from build123d import *

# Parameters (mm, degrees)
BOSS_EXTRUDE1_DEPTH = 40
SKETCH3_R           = 5
CUT_EXTRUDE1_DEPTH  = 98.082439195
FILLET1_R           = 20
CUT_EXTRUDE2_REACH  = 84.006
SKETCH4_R           = 5


with BuildPart() as part:
    # Sketch2 → Boss-Extrude1 (new body)
    with BuildSketch(Plane(origin=(0, 0, 0), x_dir=(1, 0, 0), z_dir=(0, 1, 0))):
        Polygon((-30, 0), (-30, 51.339745962), (-22.113248654, 65), (22.113248654, 65), (30, 51.339745962), (30, 0), (25, 0), (25, 50), (19.226497308, 60), (-19.226497308, 60), (-25, 50), (-25, 0), align=None)
    extrude(amount=BOSS_EXTRUDE1_DEPTH)

    # Sketch3 → Cut-Extrude1 (cut, through all)
    with BuildSketch(Plane(origin=(30, 0, 0), x_dir=(0, 0, -1), z_dir=(1, 0, 0))):
        with Locations((10, 20)):
            Circle(SKETCH3_R)
    extrude(amount=-CUT_EXTRUDE1_DEPTH, mode=Mode.SUBTRACT)

    # Fillet1
    fillet1_edges = [part.edges().sort_by_distance(p)[0] for p in [
        (27.5, 40, 0),
        (-27.5, 40, 0),
        (-27.5, 0, 0),
        (27.5, 0, 0),
    ]]
    fillet(fillet1_edges, radius=FILLET1_R - 0.0001)  # a hair under: the kernel refuses the full size

    # Sketch4 → Cut-Extrude2 (cut, up to next)
    with BuildSketch(Plane(origin=(0, 0, -65), x_dir=(-1, 0, 0), z_dir=(0, 0, -1)), mode=Mode.PRIVATE) as cut_extrude2_sk1:
        with Locations((0, 20)):
            Circle(SKETCH4_R)
    cut_extrude2_tool1 = extrude(cut_extrude2_sk1.sketch, amount=-CUT_EXTRUDE2_REACH, mode=Mode.PRIVATE) & part.part
    add(cut_extrude2_tool1.solids().sort_by_distance((0, 20, -65))[0], mode=Mode.SUBTRACT)


solid = part.part
Geometry: final body of the model. Coordinates: model frame, mm. A direction names the side the tool comes from. Round coordinates to 2 decimals unless told otherwise and drop trailing zeros. Loops run counter-clockwise (first coordinate to the right, second up) from the corner with the lowest first, then second, coordinate; pieces in that order, holes last. Notation, with made-up numbers: M 39.25,3.5 L 62.25,3.5 A24 cw 62.25,36.5 Z; hole C 8.5,-27.5 d2. An arc over 180 degrees is marked long. Put each result on its own line as item: value. Start each with the question number.
(1) Section query A-A (z = -41). Return loops of the section in (x, y).
(2) Section query B-B (x = 0). Return loops of the section in (y, z).
(3) Draft query along X for faces 3 (the face through (5, 15, -60)), 4 (the face through (-26.112, 19.72, -58.074)), 5 (the face through (0, 0, -61)). Return one class per face: +X half, -X half, draft (parallel to the pull), parting line (faces both ways), or undercut.
(4) Section query C-C (y = 17). Return loops of the section in (x, z).
(5) Contact query for flat-ended pins moving along their axis: pin 1 Ø1 at (x, y) = (-17.5, 10) entering from +Z; pin 2 Ø8 at (x, y) = (18, 8) entering from +Z; pin 3 Ø1 at (x, y) = (-21, 21.5) entering from +Z. Output: stop coordinate, or through.
(6) Section query D-D (z = -10). Return loops of the section in (x, y), then the cut area to 3 significant figures.
(7) Set-up query: faces 1 (the face through (-22.073, 19.72, -55.07)), 2 (the face through (-27.535, 6.014, -5.703)). Return all of +Z, -Z, +X, -X, +Y, -Y with unobstructed straight access to the full face (end or side cutting, diameter ignored); none if empty.
(8) Material intervals for line 1 along X through (y, z) = (18, -17.5); line 2 along Y through (x, z) = (0, -61); line 3 along Z through (x, y) = (-16.5, 12), sorted ascending. Write a range as [from, to].
Findings below:
1. outline: M -30,0 L -25,0 L -25,40 L -30,40 Z; M 25,0 L 30,0 L 30,40 L 25,40 Z
2. outline: M 0,-65 L 15,-65 L 15,-60 L 0,-60 Z; M 25,-65 L 40,-65 L 40,-60 L 25,-60 Z
3. face 3: undercut
3. face 4: -X half
3. face 5: draft
4. outline: M -30,-51.34 L -22.11,-65 L -4,-65 L -4,-60 L -19.23,-60 L -25,-50 L -25,-14 L -30,-14 Z; M -30,-6 L -25,-6 L -25,-0.23 L -30,-0.23 Z; M 4,-65 L 22.11,-65 L 30,-51.34 L 30,-14 L 25,-14 L 25,-50 L 19.23,-60 L 4,-60 Z; M 25,-6 L 30,-6 L 30,-0.23 L 25,-0.23 Z
5. pin 1: stops at z = -60
5. pin 2: stops at z = -55.2
5. pin 3: stops at z = -56.06
6. outline: M -30,2.68 L -25,2.68 L -25,15 L -30,15 Z; M -30,25 L -25,25 L -25,37.32 L -30,37.32 Z; M 25,2.68 L 30,2.68 L 30,15 L 25,15 Z; M 25,25 L 30,25 L 30,37.32 L 25,37.32 Z
6. area: 246 mm2
7. face 1: +Z, +Y, -Y
7. face 2: +Z, +X, -X, -Y
8. line 1: x = [-30, -25], [25, 30]
8. line 2: y = [0, 15], [25, 40]
8. line 3: z = [-65, -60]
